Verification items for the finished model (mm, model axes). A direction names the side the tool comes from. Round coordinates to 2 decimals unless told otherwise and drop trailing zeros. One line per question, with ' | ' between items. Start each with the question number.
Q1. Thickness scan on line 1 along Y through (x, z) = (0, 7.75); line 2 along Z through (x, y) = (27.5, 1); line 3 along Y through (x, z) = (-27, 10.25). Record the ranges inside material, lowest first. Write a range as from..to.
Q2. Cross-section at A-A (z = 3.25). State how many separate pieces and enclosed holes the cut face has, then the cut area to 3 significant figures.
Q3. Gauge pin test, flat ends, axial feed: pin 1 (0.5 mm diameter, centred on x = -5.5, y = -4.5, fed in from -Z); pin 2 (4 mm diameter, centred on x = -18, z = 13, fed in from +Y); pin 3 (11 mm diameter, centred on x = 29.5, y = 2, fed in from -Z). Record the tip position at first contact, or that the pin passes through.
Q4. Release check for a two-part mould opening along X. For faces 3 (the face through (8, -8, 11)), 4 (the face through (-8.67, -39.05, 5.42)), 5 (the face through (12, 36, 0)), 6 (the face through (-4.88, 37.18, 5.42)) record: released by +X, released by -X, zero draft, split by the parting line, or undercut.
Q5. Tool access check on faces 1 (the face through (25, 0, 8)), 2 (the face through (0, -7, 16)). Record the directions out of +Z, -Z, +X, -X, +Y, -Y that give a thin tool (end or side, any length) a straight path to the whole face; none if there is none.
from build123d import *

# Parameters (mm, degrees)
F1_R      = 40
F2_DEPTH  = 16
F3_DEPTH  = 13
F4_R      = 6.5
F5_DEPTH  = 16.001
F6_R      = 2.5
F7_DEPTH  = 16.001
F8_R      = 5
F9_R      = 37.5
F9_R_2    = 10
F9_R_3    = 5
F10_DEPTH = 11
F11_DEPTH = 5


with BuildPart() as f2:
    # F1 (on Top) → F2 (new body)
    with BuildSketch(Plane.XY):
        Circle(F1_R)
    extrude(amount=F2_DEPTH)

    # F0 (on Top) → F3 (cut)
    with BuildSketch(Plane.XY):
        Polygon((0.5, 7.4833147735), (0.5, 6.4807406984), (-0.5, 6.4807406984), (-0.5, 7.4833147735), (-2.0895980578, 7.2030257501), (-1.746697532, 6.2609142888), (-2.6863901539, 5.9188941485), (-3.0292906797, 6.8610056098), (-4.4271597759, 6.0539455166), (-3.782717585, 5.2859292156), (-4.54876203, 4.6431416082), (-5.193204221, 5.4111579093), (-6.2307406865, 4.1746701064), (-5.3624860697, 3.6733830663), (-5.8624860722, 2.807357664), (-6.730740689, 3.308644704), (-7.2828023136, 1.7918678691), (-6.2954595919, 1.6177727054), (-6.4691077722, 0.6329649529), (-7.4564504939, 0.8070601166), (-7.456450498, -0.8070600785), (-6.4691077754, -0.6329649198), (-6.2954596002, -1.6177726732), (-7.2828023228, -1.7918678319), (-6.7307407059, -3.3086446696), (-5.8624860865, -2.807357634), (-5.3624860885, -3.6733830389), (-6.2307407079, -4.1746700745), (-5.1932042487, -5.4111578827), (-4.5487620538, -4.643141585), (-3.782717612, -5.2859291963), (-4.4271598069, -6.053945494), (-3.0292907148, -6.8610055943), (-2.6863901841, -5.9188941348), (-1.746697564, -6.2609142799), (-2.0895980946, -7.2030257394), (-0.5000000128, -7.4833147727), (-0.500000011, -6.4807406976), (0.499999989, -6.4807406993), (0.4999999872, -7.4833147744), (2.0895980701, -7.2030257465), (1.7466975426, -6.2609142858), (2.686390164, -5.9188941439), (3.0292906914, -6.8610056046), (4.4271597862, -6.0539455091), (3.782717594, -5.2859292092), (4.5487620379, -4.6431416005), (5.1932042302, -5.4111579004), (6.2307406937, -4.1746700957), (5.362486076, -3.6733830572), (5.862486077, -2.807357654), (6.7307406946, -3.3086446925), (7.2828023167, -1.7918678567), (6.2954595947, -1.6177726947), (6.4691077733, -0.6329649418), (7.4564504953, -0.8070601039), (7.4564504967, 0.8070600912), (6.4691077744, 0.6329649308), (6.2954595974, 1.6177726839), (7.2828023197, 1.7918678443), (6.7307407003, 3.3086446811), (5.8624860818, 2.807357644), (5.3624860822, 3.673383048), (6.2307407008, 4.1746700851), (5.1932042394, 5.4111578916), (4.5487620458, 4.6431415927), (3.782717603, 5.2859292027), (4.4271597966, 6.0539455016), (3.0292907031, 6.8610055995), (2.686390174, 5.9188941393), (1.7466975533, 6.2609142829), (2.0895980824, 7.203025743), align=None)
    extrude(amount=F3_DEPTH, mode=Mode.SUBTRACT)

    # F4 (on Top) → F5 (cut, through all)
    with BuildSketch(Plane.XY):
        Circle(F4_R)
    extrude(amount=F5_DEPTH, mode=Mode.SUBTRACT)

    # F6 (on Top) → F7 (cut, through all)
    with BuildSketch(Plane.XY):
        with Locations((30, 0)):
            Circle(F6_R)
    extrude(amount=F7_DEPTH, mode=Mode.SUBTRACT)

    # F8
    f8_edges = [f2.edges().sort_by_distance(p)[0] for p in [
        (-40, 0, 16),
    ]]
    fillet(f8_edges, radius=F8_R)

    # F9 (on Top) → F10 (cut)
    with BuildSketch(Plane.XY):
        Circle(F9_R)
        Circle(F9_R_2, mode=Mode.SUBTRACT)
        with Locations((30, 0)):
            Circle(F9_R_3, mode=Mode.SUBTRACT)
    extrude(amount=F10_DEPTH, mode=Mode.SUBTRACT)

    # F11 (cut): a face of the model
    f11_faces = [f2.faces().sort_by_distance(p)[0] for p in [
        (25.1414213562, 0, 0),
    ]]
    extrude(f11_faces, amount=-F11_DEPTH, mode=Mode.SUBTRACT)


solid = f2.part
Determined:
1) line 1: y = -40..-37.5, -10..-6.5, 6.5..10, 37.5..40 | line 2: z = 5..16 | line 3: y = -29.51..-26.02, 26.02..29.51
2) separate pieces: 2 | enclosed holes: 2 | area: 765 mm²
3) pin 1: stops at z = 13 | pin 2: stops at y = 36.43 | pin 3: stops at z = 5
4) face 3: undercut | face 4: split by the parting line | face 5: zero draft | face 6: undercut
5) face 1: -Z | face 2: +Z, +X, -X, +Y, -Y
